```python
from build123d import *

# Parameters (mm, degrees)
SKETCH_W        = 80
SKETCH_H        = 55
PAD_DEPTH       = 6
SKETCH001_W     = 70.2
SKETCH001_H     = 50.2
POCKET_DEPTH    = 4
SKETCH002_R     = 2
PAD001_DEPTH    = 3
SKETCH003_R     = 0.9
PAD002_DEPTH    = 1
SKETCH004_W     = 3
SKETCH004_H     = 1.5
SKETCH004_H_2   = 3
POCKET001_DEPTH = 6
SKETCH005_W     = 3
SKETCH005_H     = 5
SKETCH005_H_2   = 21
POCKET002_DEPTH = 3
SKETCH006_W     = 5
SKETCH006_H     = 2
POCKET003_DEPTH = 1
SKETCH007_W     = 5
SKETCH007_H     = 2
POCKET004_DEPTH = 1


with BuildPart() as part:
    # Sketch → Pad (new body)
    with BuildSketch(Plane.XY):
        with Locations((3, 0)):
            Rectangle(SKETCH_W, SKETCH_H)
    extrude(amount=PAD_DEPTH)

    # Sketch001 (on Face6 of Pad) → Pocket (cut)
    with BuildSketch(Plane.XY.offset(6)):
        Rectangle(SKETCH001_W, SKETCH001_H)
    extrude(amount=-POCKET_DEPTH, mode=Mode.SUBTRACT)

    # Sketch002 (on Face11 of Pocket) → Pad001 (join)
    with BuildSketch(Plane.XY.offset(2)):
        with Locations((-32.5, 22.5)):
            Circle(SKETCH002_R)
        with Locations((32.5, 22.5)):
            Circle(SKETCH002_R)
        with Locations((-32.5, -22.5)):
            Circle(SKETCH002_R)
        with Locations((32.5, -22.5)):
            Circle(SKETCH002_R)
    extrude(amount=PAD001_DEPTH)

    # Sketch003 (on Face19 of Pad001) → Pad002 (join)
    with BuildSketch(Plane.XY.offset(5)):
        with Locations((-32.5, 22.5)):
            Circle(SKETCH003_R)
        with Locations((32.5, 22.5)):
            Circle(SKETCH003_R)
        with Locations((-32.5, -22.5)):
            Circle(SKETCH003_R)
        with Locations((32.5, -22.5)):
            Circle(SKETCH003_R)
    extrude(amount=PAD002_DEPTH)

    # Sketch004 (on Face5 of Pad002) → Pocket001 (cut)
    with BuildSketch(Plane.XY.offset(6)):
        with Locations((39, 16.75)):
            Rectangle(SKETCH004_W, SKETCH004_H)
        with Locations((39, 9.5)):
            Rectangle(SKETCH004_W, SKETCH004_H_2)
        with Locations((39, 1.5)):
            Rectangle(SKETCH004_W, SKETCH004_H_2)
        with Locations((39, -5.75)):
            Rectangle(SKETCH004_W, SKETCH004_H)
        with Locations((39, -14.75)):
            Rectangle(SKETCH004_W, SKETCH004_H)
        with Locations((39, -21.25)):
            Rectangle(SKETCH004_W, SKETCH004_H)
    extrude(amount=-POCKET001_DEPTH, mode=Mode.SUBTRACT)

    # Sketch005 (on Face4 of Pocket001) → Pocket002 (cut)
    with BuildSketch(Plane(origin=(0, 0, 0), x_dir=(1, 0, 0), z_dir=(0, 0, -1))):
        with Locations((39, 18)):
            Rectangle(SKETCH005_W, SKETCH005_H)
        with Locations((39, -5.5)):
            Rectangle(SKETCH005_W, SKETCH005_H_2)
    extrude(amount=-POCKET002_DEPTH, mode=Mode.SUBTRACT)

    # Sketch006 (on Face6 of Pocket002) → Pocket003 (cut)
    with BuildSketch(Plane.XZ.offset(27.5)):
        with Locations((-18.5, 3)):
            Rectangle(SKETCH006_W, SKETCH006_H)
        with Locations((18.5, 3)):
            Rectangle(SKETCH006_W, SKETCH006_H)
    extrude(amount=-POCKET003_DEPTH, mode=Mode.SUBTRACT)

    # Sketch007 (on Face1 of Pocket003) → Pocket004 (cut)
    with BuildSketch(Plane(origin=(0, 27.5, 0), x_dir=(-1, 0, 0), z_dir=(0, 1, 0))):
        with Locations((-18.5, 3)):
            Rectangle(SKETCH007_W, SKETCH007_H)
        with Locations((18.5, 3)):
            Rectangle(SKETCH007_W, SKETCH007_H)
    extrude(amount=-POCKET004_DEPTH, mode=Mode.SUBTRACT)


solid = part.part
```
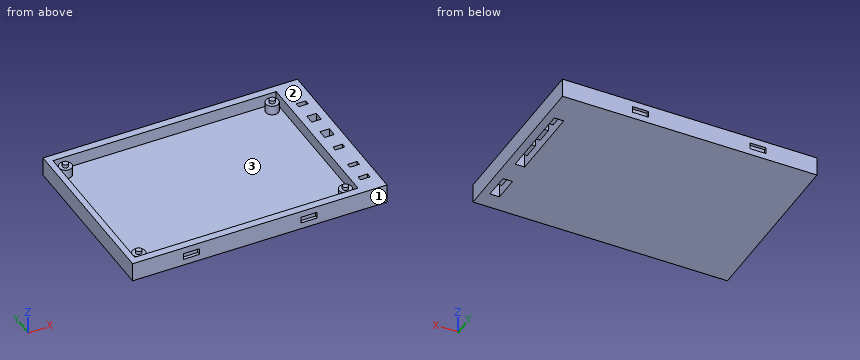
Design review of the part built by this model. Coordinates are the model's own, in mm. Face numbers are marked on the shaded views. Coordinates: 2 decimals unless noted, no trailing zeros. Order: outer loops, then holes, each group sorted by start corner. A loop starts at its lowest first (then second) coordinate and runs counter-clockwise, first axis right, second up. Notation, with made-up numbers: (10.25, 12) -> (49.25, 12) arc R29 cw to (49.25, 50) -> close; hole circle Ø10 at (68, 40). An arc over 180 degrees is marked (long way). One line per item, written item: value. Start each with the question number.
Q1. Take a section at C-C, the plane y = 18.5. State the section outline as (x, z) points.
Q2. Insertion check: pin 1 Ø1.5 at (x, y) = (-18.5, -16) entering from +Z; pin 2 Ø0.9 at (x, y) = (39, 5) entering from -Z. Each pin has a flat end and moves straight along its axis. Give the tip position at first contact, or say it passes through.
Q3. Take a section at B-B, the plane x = 32.5. State the section outline as (y, z) points, then the cut area to 3 significant figures.
Q4. For probe 1 along X at (y, z) = (9, 5.75); probe 2 along X at (y, z) = (-10.5, 3.25); probe 3 along Y at (x, z) = (-2, 2.45), list the stretches that pass through material, from the lowest coordinate up.
Q5. Take a section at D-D, the plane y = -18. State the section outline as (x, z) points, then the cut area to 3 significant figures.
Q6. Mouldability with a two-part tool opening along Y and no side actions: class the marked faces 1, 2 and 3 as pulls with the +Y half, pulls with the -Y half, needs draft (parallel to the pull), parting line crosses it, or undercut.
Q7. Take a section at A-A, the plane y = 2. State the section outline as (x, z) points, then the cut area to 3 significant figures.
Values follow:
1. outline: (-37, 0) -> (43, 0) -> (43, 6) -> (35.1, 6) -> (35.1, 2) -> (-35.1, 2) -> (-35.1, 6) -> (-37, 6) -> close
2. pin 1: stops at z = 2
2. pin 2: stops at z = 3
3. outline: (-27.5, 0) -> (27.5, 0) -> (27.5, 6) -> (25.1, 6) -> (25.1, 2) -> (24.5, 2) -> (24.5, 5) -> (23.4, 5) -> (23.4, 6) -> (21.6, 6) -> (21.6, 5) -> (20.5, 5) -> (20.5, 2) -> (-20.5, 2) -> (-20.5, 5) -> (-21.6, 5) -> (-21.6, 6) -> (-23.4, 6) -> (-23.4, 5) -> (-24.5, 5) -> (-24.5, 2) -> (-25.1, 2) -> (-25.1, 6) -> (-27.5, 6) -> close
3. area: 157 mm2
4. probe 1: x = -37 to -35.1, 35.1 to 37.5, 40.5 to 43
4. probe 2: x = -37 to -35.1, 35.1 to 43
4. probe 3: y = -27.5 to -25.1, 25.1 to 27.5
5. outline: (-37, 0) -> (37.5, 0) -> (37.5, 3) -> (40.5, 3) -> (40.5, 0) -> (43, 0) -> (43, 6) -> (35.1, 6) -> (35.1, 2) -> (-35.1, 2) -> (-35.1, 6) -> (-37, 6) -> close
5. area: 190 mm2
6. face 1: pulls with the -Y half
6. face 2: needs draft
6. face 3: undercut
7. outline: (-37, 0) -> (37.5, 0) -> (37.5, 6) -> (35.1, 6) -> (35.1, 2) -> (-35.1, 2) -> (-35.1, 6) -> (-37, 6) -> close; (40.5, 0) -> (43, 0) -> (43, 6) -> (40.5, 6) -> close
7. area: 181 mm2
